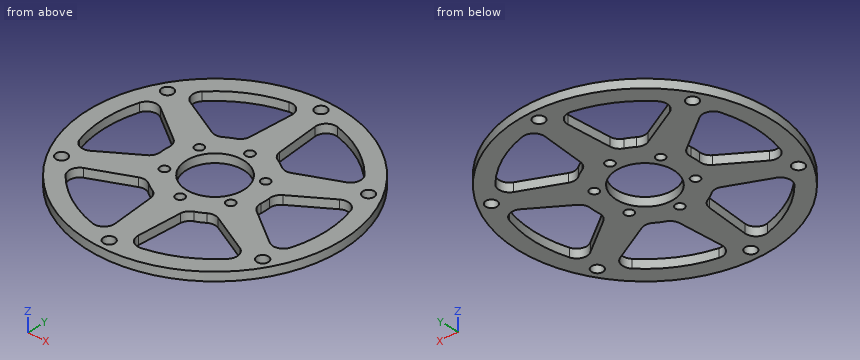
Autodesk Inventor part; units mm, degrees
ref_plane "YZ Plane" through (0, 0, 0) normal (1, 0, 0) x (0, 1, 0)
ref_plane "XZ Plane" through (0, 0, 0) normal (0, 1, 0) x (-1, 0, 0)
ref_plane "XY Plane" through (0, 0, 0) normal (0, 0, 1) x (1, 0, 0)
sketch "Sketch1" plane through (0, 0, 0) normal (0, 0, 1) x (1, 0, 0)
  circle A0 centre (0, 0) radius 16.5
  circle A1 centre (0, 0) radius 73
  point P0 (0, 66.675)
  point P1 (-57.7422, 33.3375)
  point P2 (-57.7422, -33.3375)
  point P3 (0, -66.675)
  point P4 (57.7422, -33.3375)
  point P5 (57.7422, 33.3375)
  point P6 (0, 22)
  point P7 (-19.0526, 11)
  point P8 (-19.0526, -11)
  point P9 (0, -22)
  point P10 (19.0526, -11)
  point P11 (19.0526, 11)
  dimension "d0" = 66.675
  dimension "d3" = 360
  dimension "d9" = 33
  dimension "d20" = 22
  dimension "d23" = 360
  dimension "d25" = 146
extrude "Extrusion2" add sketch "Sketch1" along normal blind 5
hole "Hole2" at (0, 66.675, 0) at (-57.7422, 33.3375, 0) at (-57.7422, -33.3375, 0) at (0, -66.675, 0) at (57.7422, -33.3375, 0) at (57.7422, 33.3375, 0) direction (0, 0, 1) diameter 6.5 end through all
hole "Hole3" at (0, 22, 0) at (-19.0526, 11, 0) at (-19.0526, -11, 0) at (0, -22, 0) at (19.0526, 11, 0) at (19.0526, -11, 0) direction (0, 0, 1) diameter 5 end through all
sketch "Sketch4" plane through (0, 0, 5) normal (0, 0, 1) x (1, 0, 0)
  circle A0 centre (0, 0) radius 28.9422 construction
  line L0 (0, 0) -> (58.5803, 0) construction
  circle A1 centre (-57.7422, 33.3375) radius 3.25 construction
  circle A2 centre (0, 66.675) radius 3.25 construction
  line L1 (-57.7422, 33.3375) -> (0, 66.675) construction
  circle A3 centre (0, 0) radius 16.5 construction
  circle A4 centre (-19.0526, 11) radius 2.5 construction
  circle A5 centre (0, 22) radius 2.5 construction
  line L2 (-19.0526, 11) -> (0, 22) construction
  circle A6 centre (0, 0) radius 63.4652 construction
  arc A7 (-6.0622, 63.175) -> (-51.6801, 36.8375) centre (0, 0) ccw
  line L3 (-9.5263, 16.5) -> (-21.2308, 36.7728) construction
  line L4 (-8.8547, 27.5544) -> (-19.4354, 21.4456) construction
  line L5 (-8.8547, 27.5544) -> (-6.0622, 63.175)
  line L6 (-19.4354, 21.4456) -> (-51.6801, 36.8375)
  arc A8 (-8.8547, 27.5544) -> (-19.4354, 21.4456) centre (0, 0) ccw
  point P0 (-14.1451, 24.5)
  dimension "d60" = 7
  dimension "d61" = 7
extrude "Extrusion4" cut sketch "Sketch4" against normal blind 10
fillet "Fillet1" radius 6 4 edges at (-51.6801, 36.8375, 2.5) (-6.0622, 63.175, 2.5) (-8.8547, 27.5544, 2.5) (-19.4354, 21.4456, 2.5)
pattern_circular "Circular Pattern1" count 6 over 360 about axis through (0, 0, -10) along (0, 0, 1) of "Extrusion4", "Fillet1"
equation "\"d61\" = d60"
properties part number "SprocketHubPlate_plasmacut"
Source: CAD feature listing. Evaluate the final solid. Frame: model axes, mm. Give positions to 0.01 mm unless a question says otherwise; leave off trailing zeros. Write each loop counter-clockwise with the first axis right and the second up, starting at its lowest first coordinate (ties: lowest second). Pieces come first, ordered by that corner, then holes. Notation, with made-up numbers: M 52.5,54.5 L 91.5,54.5 A14 cw 91.5,75.5 Z; hole C 59,-13.75 d1. An arc over 180 degrees is marked long. Answer as a JSON object with one key per item and string values.
Q1. Cut plane C-C, the plane x = -33.5. Return the cut outline in (y, z).
Geometry check:
{"outline": "M -64.86,0 L -53.9,0 L -53.9,5 L -64.86,5 Z; M -28.16,0 L -9.69,0 L -9.69,5 L -28.16,5 Z; M 9.69,0 L 28.16,0 L 28.16,5 L 9.69,5 Z; M 53.9,0 L 64.86,0 L 64.86,5 L 53.9,5 Z"}
Q2. Cut plane D-D, the plane y = -51. Return the cut outline in (x, z).
Geometry check:
{"outline": "M -52.23,0 L -37.77,0 L -37.77,5 L -52.23,5 Z; M -7.02,0 L 7.02,0 L 7.02,5 L -7.02,5 Z; M 37.77,0 L 52.23,0 L 52.23,5 L 37.77,5 Z"}
Q3. Ray query, line 1 along X through (y, z) = (-20, 3.1); line 2 along Y through (x, z) = (-30, 0.35); line 3 along X through (y, z) = (-43.5, 3.15). Return the intervals inside material, ascending.
Geometry check:
{"line 1": "x = -70.21 to -60.11, -48.52 to -1.5, 1.5 to 48.52, 60.11 to 70.21", "line 2": "y = -66.55 to -55.93, -26.49 to -6.91, 6.91 to 26.49, 55.93 to 66.55", "line 3": "x = -58.62 to -46.21, -7.6 to 7.6, 46.21 to 58.62"}
Q4. Cut plane A-A, the plane y = 0. Return the cut outline in (x, z).
Geometry check:
{"outline": "M -73,0 L -63.47,0 L -63.47,5 L -73,5 Z; M -28.94,0 L -16.5,0 L -16.5,5 L -28.94,5 Z; M 16.5,0 L 28.94,0 L 28.94,5 L 16.5,5 Z; M 63.47,0 L 73,0 L 73,5 L 63.47,5 Z"}
Q5. Contact query for flat-ended pins moving along their axis: P1, Ø2, axis at x = -50.5, z = 1, coming from the +Y side; P2, Ø1.5, axis at x = -41, z = 0.5, coming from the -Y side. Output: stop coordinate, or through.
Geometry check:
{"P1": "stops at y = 53.65", "P2": "stops at y = -60.9"}
Q6. Cut plane B-B, the plane x = 0. Return the cut outline in (y, z) (3 decimals).
Geometry check:
{"outline": "M -73,0 L -69.925,0 L -69.925,5 L -73,5 Z; M -63.425,0 L -24.5,0 L -24.5,5 L -63.425,5 Z; M -19.5,0 L -16.5,0 L -16.5,5 L -19.5,5 Z; M 16.5,0 L 19.5,0 L 19.5,5 L 16.5,5 Z; M 24.5,0 L 63.425,0 L 63.425,5 L 24.5,5 Z; M 69.925,0 L 73,0 L 73,5 L 69.925,5 Z"}
